Input: part model. Units: mm. Frame: model coordinates. Give positions to 0.01 mm unless a question says otherwise; leave off trailing zeros. Write each loop counter-clockwise with the first axis right and the second up, starting at its lowest first coordinate (ties: lowest second). Pieces come first, ordered by that corner, then holes.
```python
from build123d import *

# Parameters (mm, degrees)
CROQUIS2_R                 = 37.79
SALIENTE_EXTRUIR1_DEPTH    = 5
CROQUIS4_W                 = 6
CROQUIS4_H                 = 25
SALIENTE_EXTRUIR3_DEPTH    = 2.5
CROQUIS5_R                 = 1.25
CORTAR_EXTRUIR1_DEPTH      = 21.29
CORTAR_EXTRUIR1_DEPTH_BACK = 56.29
REDONDEO1_R                = 5
CORTAR_EXTRUIR2_START      = 50
CROQUIS6_R                 = 2
CORTAR_EXTRUIR2_DEPTH      = 17
MATRIZC1_COUNT             = 4
SALIENTE_EXTRUIR5_DEPTH    = 5


with BuildPart() as part:
    # Croquis2 → Saliente-Extruir1 (new body)
    with BuildSketch(Plane(origin=(0, 0, 0), x_dir=(1, 0, 0), z_dir=(0, 1, 0))):
        Circle(CROQUIS2_R)
        with BuildLine():
            Line((-12.586494468, 15), (12.586494468, 15))
            Line((12.586494468, 15), (23.005368551, 27.416730619))
            ThreePointArc((23.005368551, 27.416730619), (35.79, 0), (23.005368551, -27.416730619))
            Line((23.005368551, -27.416730619), (12.586494468, -15))
            Line((12.586494468, -15), (-12.586494468, -15))
            Line((-12.586494468, -15), (-23.005368551, -27.416730619))
            ThreePointArc((-23.005368551, -27.416730619), (-35.79, 0), (-23.005368551, 27.416730619))
            Line((-23.005368551, 27.416730619), (-12.586494468, 15))
        make_face(mode=Mode.SUBTRACT)
        with BuildLine():
            Line((-11.420725322, 17.5), (-21.034063882, 28.956730765))
            ThreePointArc((-21.034063882, 28.956730765), (0, 35.79), (21.034063882, 28.956730765))
            Line((21.034063882, 28.956730765), (11.420725322, 17.5))
            Line((11.420725322, 17.5), (-11.420725322, 17.5))
        make_face(mode=Mode.SUBTRACT)
        with BuildLine():
            ThreePointArc((21.034063882, -28.956730765), (0, -35.79), (-21.034063882, -28.956730765))
            Line((-21.034063882, -28.956730765), (-11.420725322, -17.5))
            Line((-11.420725322, -17.5), (11.420725322, -17.5))
            Line((11.420725322, -17.5), (21.034063882, -28.956730765))
        make_face(mode=Mode.SUBTRACT)
    extrude(amount=SALIENTE_EXTRUIR1_DEPTH)

    # Croquis4 → Saliente-Extruir3 (add)
    with BuildSketch(Plane.XY.offset(15)):
        with Locations((0, 12.5)):
            Rectangle(CROQUIS4_W, CROQUIS4_H)
    saliente_extruir3 = extrude(amount=SALIENTE_EXTRUIR3_DEPTH)

    # Simetría1: Saliente-Extruir3 across plane
    add(saliente_extruir3.mirror(Plane.XY))

    # Croquis5 → Cortar-Extruir1 (cut, two sides)
    with BuildSketch(Plane(origin=(0, 0, -17.5), x_dir=(-1, 0, 0), z_dir=(0, 0, -1))) as cortar_extruir1_sk:
        with Locations((0, 23)):
            Circle(CROQUIS5_R)
    extrude(amount=CORTAR_EXTRUIR1_DEPTH, mode=Mode.SUBTRACT)
    extrude(cortar_extruir1_sk.sketch, amount=-CORTAR_EXTRUIR1_DEPTH_BACK, mode=Mode.SUBTRACT)

    # Redondeo1
    redondeo1_edges = [part.edges().sort_by_distance(p)[0] for p in [
        (-11.420725322, 2.5, -17.5),
        (11.420725322, 2.5, -17.5),
        (11.420725322, 2.5, 17.5),
        (-11.420725322, 2.5, 17.5),
    ]]
    fillet(redondeo1_edges, radius=REDONDEO1_R)

    # Croquis6 → Cortar-Extruir2 (cut)
    with BuildSketch(Plane.XY.offset(CORTAR_EXTRUIR2_START)):
        with Locations((0, 2.5)):
            Circle(CROQUIS6_R)
    cortar_extruir2 = extrude(amount=-CORTAR_EXTRUIR2_DEPTH, mode=Mode.SUBTRACT)

    # MatrizC1: Cortar-Extruir2 ×4 about axis
    matrizc1_axis = Axis((0, 0, 0), (0, -1, 0))
    for i in range(1, MATRIZC1_COUNT):
        add(cortar_extruir2.rotate(matrizc1_axis, i * 360 / MATRIZC1_COUNT), mode=Mode.SUBTRACT)

    # Croquis8 → Saliente-Extruir5 (add)
    with BuildSketch(Plane(origin=(0, 5, 0), x_dir=(1, 0, 0), z_dir=(0, 1, 0))):
        with BuildLine():
            Line((-14.684243546, -17.5), (-12.586494468, -15))
            Line((-12.586494468, -15), (-32.494985767, -15))
            ThreePointArc((-32.494985767, -15), (-31.881892303, -16.26250421), (-31.219770979, -17.5))
            Line((-31.219770979, -17.5), (-14.684243546, -17.5))
        make_face()
    extrude(amount=-SALIENTE_EXTRUIR5_DEPTH)


solid = part.part
```
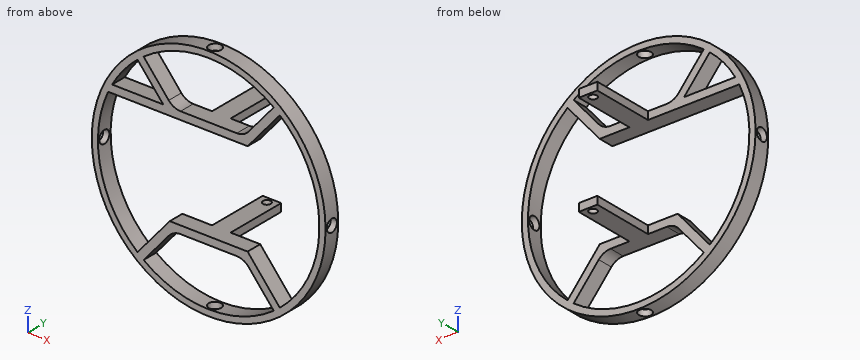
Q1. Section C-C, the plane x = 0. Give the number of separate pieces and of enclosed holes in the cut face, then the cut area to 4 significant figures.
Q2. Section B-B, the plane y = 23. Return the cut outline in (x, z), then the cut area to 3 significant figures.
Q3. Section A-A, the plane y = 18.25. Return the cut outline in (x, z), then the cut area to 3 significant figures.
Q4. Material intervals for line 1 along Y through (x, z) = (36.4, 0); line 2 along Y through (x, z) = (-20.5, 31); line 3 along Z through (x, y) = (1.5, 1.5), sorted ascending.
Q5. Section D-D, the plane z = 31. Return the cut outline in (x, y), then the cut area to 3 significant figures.
Q6. Pin query (flat end, axial travel): pin 1 (5.5 mm diameter, centred on x = -26.5, y = 2, fed in from +Z); pin 2 (6 mm diameter, centred on x = -28.5, z = -22.5, fed in from +Y); pin 3 (10 mm diameter, centred on y = 17, z = -10.5, fed in from -X). Return the tip coordinate at first contact, or that it passes through.
Solutions:
1. separate pieces: 8
1. enclosed holes: 0
1. area: 116.5 mm2
2. outline: (-3, -17.5) - (-1.25, -17.5) - (-1.25, -15) - (-3, -15) - close; (-3, 15) - (-1.25, 15) - (-1.25, 17.5) - (-3, 17.5) - close; (1.25, -17.5) - (3, -17.5) - (3, -15) - (1.25, -15) - close; (1.25, 15) - (3, 15) - (3, 17.5) - (1.25, 17.5) - close
2. area: 17.5 mm2
3. outline: (-3, -17.5) - (3, -17.5) - (3, -15) - (-3, -15) - close; (-3, 15) - (3, 15) - (3, 17.5) - (-3, 17.5) - close
3. area: 30.0 mm2
4. line 1: y = 0 to 0.5, 4.5 to 5
4. line 2: y = 0 to 5
4. line 3: z = -17.5 to -15, 15 to 17.5
5. outline: (-21.61, 0) - (-17.89, 0) - (-17.89, 5) - (-21.61, 5) - close; (17.89, 0) - (21.61, 0) - (21.61, 5) - (17.89, 5) - close
5. area: 37.3 mm2
6. pin 1: stops at z = 29.39
6. pin 2: stops at y = 5
6. pin 3: stops at x = -3
